Verification items for the finished model (mm, model axes). Face numbers are marked on the shaded views. A direction names the side the tool comes from. Coordinates: 2 decimals unless noted, no trailing zeros. Order: outer loops, then holes, each group sorted by start corner. A loop starts at its lowest first (then second) coordinate and runs counter-clockwise, first axis right, second up. Notation, with made-up numbers: M 53.5,-37.75 L 83.5,-37.75 A13 cw 83.5,-33.75 Z; hole C 77,31 d1. An arc over 180 degrees is marked long. Return JSON: item names as keys, results as strings. Group by question number.
Q1. Mould release check, pull along Y, two halves, no side actions. Record for the marked faces 3, 4 and 5: pulls with the +Y half, pulls with the -Y half, needs draft (parallel to the pull), parting line crosses it, or undercut.
Q2. Thickness scan on probe 1 along Y at (x, z) = (0, 3.85); probe 2 along Y at (x, z) = (0, 0). Record the ranges inside material, lowest first.
Q3. Section check D-D, the plane x = -11.25. Enter the section's corners in (y, z), then the cut area to 3 significant figures.
Q4. Section check A-A, the plane y = 0. Enter the section's corners in (x, z).
Q5. Access from +Z, -Z, +X, -X, +Y, -Y to the whole of each face (thin tool, end or side, straight path). Record for the marked faces 1 and 2.
Q6. Go/stop test with flat-tipped pins: pin 1 Ø4 at (y, z) = (3.5, -3) entering from -X; pin 2 Ø4 at (x, z) = (5, -3) entering from +Y; pin 3 Ø2 at (x, z) = (-10.5, 0.5) entering from -Y. Record where each tip stops, or that it passes through.
Autodesk Inventor part; units mm, degrees
ref_plane "YZ Plane" through (0, 0, 0) normal (1, 0, 0) x (0, 1, 0)
ref_plane "XZ Plane" through (0, 0, 0) normal (0, 1, 0) x (-1, 0, 0)
ref_plane "XY Plane" through (0, 0, 0) normal (0, 0, 1) x (1, 0, 0)
sketch "Sketch1" plane through (0, 0, 0) normal (0, 0, 1) x (1, 0, 0)
  line L0 (-20.0025, 0) -> (20.0025, 0)
  line L1 (0, -20.0025) -> (0, 20.0025)
  circle A0 centre (0, 0) radius 14.2875
  circle A1 centre (0, 0) radius 6.35
  dimension "d0" = 12.7
  dimension "d1" = 28.575
extrude "Base" add sketch "Sketch1" along normal mid plane 7.9375 contours A1 L1 A0 L0 | L0 A0 L1 A1 | A1 L0 A0 L1 | L1 A0 L0 A1
sketch "Sketch3" plane through (0, 0, 3.9688) normal (0, 0, 1) x (1, 0, 0)
  circle A0 centre (0, 0) radius 14.2875
  circle A1 centre (0, 0) radius 6.35
  circle A2 centre (0, 0) radius 7.9375
  circle A3 centre (0, 0) radius 11.9062
  circle A4 centre (0, 0) radius 6.35
  circle A5 centre (0, 0) radius 14.2875
  dimension "d7" = 1.5875
  dimension "d8" = 2.3813
extrude "Cutaway" cut sketch "Sketch3" against normal blind 0.3969 contours A3
mirror "Mirror2" about plane through (0, 0, 0) normal (0, 0, 1) of "Cutaway"
properties part number "bearing" material "Steel"
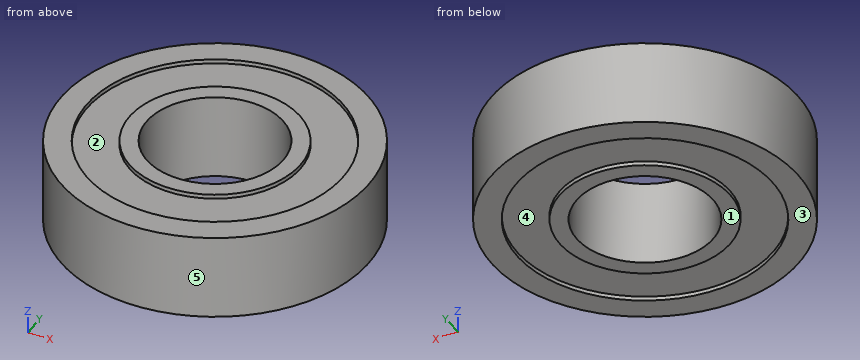
Numbers:
{
 "1": {"face 3": "needs draft", "face 4": "undercut", "face 5": "parting line crosses it"},
 "2": {"probe 1": "y = -14.29 to -11.91, -7.94 to -6.35, 6.35 to 7.94, 11.91 to 14.29", "probe 2": "y = -14.29 to -6.35, 6.35 to 14.29"},
 "3": {"outline": "M -8.81,-3.97 L -3.9,-3.97 L -3.9,-3.57 L 3.9,-3.57 L 3.9,-3.97 L 8.81,-3.97 L 8.81,3.97 L 3.9,3.97 L 3.9,3.57 L -3.9,3.57 L -3.9,3.97 L -8.81,3.97 Z", "area": "134 mm2"},
 "4": {"outline": "M -14.29,-3.97 L -11.91,-3.97 L -11.91,-3.57 L -7.94,-3.57 L -7.94,-3.97 L -6.35,-3.97 L -6.35,3.97 L -7.94,3.97 L -7.94,3.57 L -11.91,3.57 L -11.91,3.97 L -14.29,3.97 Z; M 6.35,-3.97 L 7.94,-3.97 L 7.94,-3.57 L 11.91,-3.57 L 11.91,-3.97 L 14.29,-3.97 L 14.29,3.97 L 11.91,3.97 L 11.91,3.57 L 7.94,3.57 L 7.94,3.97 L 6.35,3.97 Z"},
 "5": {"face 1": "-Z, +X, -X, +Y, -Y", "face 2": "+Z"},
 "6": {"pin 1": "stops at x = -14.21", "pin 2": "stops at y = 13.97", "pin 3": "stops at y = -10.67"}
}
